from build123d import *

# Parameters (mm, degrees)
BOSS_EXTRUDE1_DEPTH            = 3.175
SKETCH2_W                      = 31.75
SKETCH2_H                      = 82.55
CUT_EXTRUDE1_DEPTH             = 4.175
FILLET1_R                      = 3.175
F_1_4_0_25_DIAMETER_HOLE1_D    = 6.35
F_1_4_CLEARANCE_HOLE1_D        = 6.7564
F_5_16_0_3125_DIAMETER_HOLE1_D = 7.9375
CUT_EXTRUDE2_DEPTH             = 4.175
FILLET2_R                      = 6.35
SKETCH12_W                     = 31.75
SKETCH12_H                     = 50.8
CUT_EXTRUDE3_DEPTH             = 4.175
FILLET3_R                      = 3.175


with BuildPart() as part:
    # Sketch1 → Boss-Extrude1 (new body)
    with BuildSketch(Plane(origin=(0, 0, 0), x_dir=(1, 0, 0), z_dir=(0, 1, 0))):
        with BuildLine():
            Line((-260.839523021, 465.231358695), (-482.578348021, 61.34030281))
            Line((-482.578348021, 61.34030281), (-458.5319125, 48.13865281))
            ThreePointArc((-458.5319125, 48.13865281), (-449.57100781, 39.462418136), (-446.278, 27.432))
            Line((-446.278, 27.432), (-446.278, 0))
            Line((-446.278, 0), (446.278, 0))
            Line((446.278, 0), (446.278, 27.432))
            ThreePointArc((446.278, 27.432), (449.57100781, 39.462418136), (458.5319125, 48.13865281))
            Line((458.5319125, 48.13865281), (482.578348021, 61.34030281))
            Line((482.578348021, 61.34030281), (260.839523021, 465.231358695))
            Line((260.839523021, 465.231358695), (236.7930875, 452.029708695))
            ThreePointArc((236.7930875, 452.029708695), (213.394581864, 452.407369315), (201.803, 472.736361505))
            Line((201.803, 472.736361505), (201.803, 500.168361505))
            Line((201.803, 500.168361505), (-201.803, 500.168361505))
            Line((-201.803, 500.168361505), (-201.803, 472.736361505))
            ThreePointArc((-201.803, 472.736361505), (-213.394581864, 452.407369315), (-236.7930875, 452.029708695))
            Line((-236.7930875, 452.029708695), (-260.839523021, 465.231358695))
        make_face()
    extrude(amount=BOSS_EXTRUDE1_DEPTH)

    # Sketch2 → Cut-Extrude1 (cut, through all)
    with BuildSketch(Plane(origin=(0, 3.175, 0), x_dir=(1, 0, 0), z_dir=(0, 1, 0))):
        with Locations((-304.8, 41.275)):
            Rectangle(SKETCH2_W, SKETCH2_H)
        with Locations((304.8, 41.275)):
            Rectangle(SKETCH2_W, SKETCH2_H)
    extrude(amount=-CUT_EXTRUDE1_DEPTH, mode=Mode.SUBTRACT)

    # Fillet1
    fillet1_edges = [part.edges().sort_by_distance(p)[0] for p in [
        (-288.925, 1.5875, -82.55),
        (-288.925, 1.5875, 0),
        (-320.675, 1.5875, 0),
        (-320.675, 1.5875, -82.55),
        (288.925, 1.5875, 0),
        (288.925, 1.5875, -82.55),
        (320.675, 1.5875, -82.55),
        (320.675, 1.5875, 0),
    ]]
    fillet(fillet1_edges, radius=FILLET1_R)

    # 1/4 (0.25) Diameter Hole1 (through all)
    with Locations(Plane(origin=(0, 3.175, 0), x_dir=(1, 0, 0), z_dir=(0, 1, 0))):
        with Locations((-465.394777961, 66.250083744), (-272.870715461, 416.927268429), (-177.8, 487.468361505), (465.394777961, 66.250083744), (272.870715461, 416.927268429), (177.8, 487.468361505)):
            Hole(F_1_4_0_25_DIAMETER_HOLE1_D / 2)

    # 1/4 Clearance Hole1 (through all)
    with Locations(Plane(origin=(0, 3.175, 0), x_dir=(1, 0, 0), z_dir=(0, 1, 0))):
        with Locations((0, 224.282), (-376.682, 50.8), (-185.674, 398.526), (376.682, 50.8), (185.674, 398.526)):
            Hole(F_1_4_CLEARANCE_HOLE1_D / 2)

    # 5/16 (0.3125) Diameter Hole1 (through all)
    with Locations(Plane(origin=(0, 3.175, 0), x_dir=(1, 0, 0), z_dir=(0, 1, 0))):
        with Locations((-254, 50.8), (-114.3, 449.368361505), (254, 50.8), (114.3, 449.368361505)):
            Hole(F_5_16_0_3125_DIAMETER_HOLE1_D / 2)

    # Sketch11 → Cut-Extrude2 (cut, through all)
    with BuildSketch(Plane(origin=(0, 3.175, 0), x_dir=(1, 0, 0), z_dir=(0, 1, 0))):
        Polygon((0, 256.032), (159.899523893, 417.618361505), (-159.899523893, 417.618361505), align=None)
    extrude(amount=-CUT_EXTRUDE2_DEPTH, mode=Mode.SUBTRACT)

    # Fillet2
    fillet2_edges = [part.edges().sort_by_distance(p)[0] for p in [
        (0, 1.5875, -256.032),
        (-159.899523893, 1.5875, -417.618361505),
        (159.899523893, 1.5875, -417.618361505),
    ]]
    fillet(fillet2_edges, radius=FILLET2_R)

    # Sketch12 → Cut-Extrude3 (cut, through all)
    with BuildSketch(Plane(origin=(0, 3.175, 0), x_dir=(1, 0, 0), z_dir=(0, 1, 0))):
        with Locations((0, 474.768361505)):
            Rectangle(SKETCH12_W, SKETCH12_H)
    extrude(amount=-CUT_EXTRUDE3_DEPTH, mode=Mode.SUBTRACT)

    # Fillet3
    fillet3_edges = [part.edges().sort_by_distance(p)[0] for p in [
        (-15.875, 1.5875, -449.368361505),
        (-15.875, 1.5875, -500.168361505),
        (15.875, 1.5875, -500.168361505),
        (15.875, 1.5875, -449.368361505),
    ]]
    fillet(fillet3_edges, radius=FILLET3_R)


solid = part.part
CAD build for the part. Positions are in the model's coordinates, mm. A direction names the side the tool comes from. Give positions to 0.01 mm unless a question says otherwise; leave off trailing zeros. Loops run counter-clockwise (first coordinate to the right, second up) from the corner with the lowest first, then second, coordinate; pieces in that order, holes last. Notation, with made-up numbers: M 18,-11 L 33,-11 A31 cw 33,18 Z; hole C 69.5,-28 d4. An arc over 180 degrees is marked long. Answer in a Markdown table with one row per item. Add a question column.
Item 1: Band-saw the part on C-C on y = 0.6. Give the number of separate pieces and of enclosed holes in the cut face, then the cut area to 3 significant figures.
Item 2: Mould opens along X. For faces 1 (the face through (213.691, 1.565, -452.235)), 2 (the face through (-7, 3.175, -198)), 3 (the face through (-213.101, 1.565, -452.584)), 4 (the face through (373.26, 1.57, -260.46)) say: +X half, -X half, draft (parallel to the pull), parting line (faces both ways), or undercut.
Item 3: Tool access for faces 5 (the face through (-7, 0, -198)), 6 (the face through (-77.868, 1.61, -334.721)): list every direction of +Z, -Z, +X, -X, +Y, -Y with a clear straight run to the whole face (end or side of a thin tool).
Item 4: Drop flat-ended pins along their axis: P1, Ø1.6, axis at x = -298.5, y = 2, coming from the +Z side; P2, Ø1.6, axis at y = 1.5, z = -484, coming from the +X side. Give the stop position or say it passes through.
Item 5: Band-saw the part on B-B on x = -34. Give the cut face in (y, z) (3 decimals), then the cut area to 3 significant figures.
Item 6: Band-saw the part on A-A on z = -279. Give the cut face in (x, y) (3 decimals).
Item 7: Probe probe 1 along Z at (x, y) = (45, 2.75); probe 2 along Z at (x, y) = (114.3, 2.3); probe 3 along X at (y, z) = (1.35, -390.5). List the from-to ranges inside material, lowest first.
Item 8: Band-saw the part on D-D on z = -433.5. Give the cut face in (x, y) (3 decimals), then the cut area to 3 significant figures.
Reply:
| question | item | result |
|---|---|---|
| 1 | separate pieces | 1 |
| 1 | enclosed holes | 16 |
| 1 | area | 336,000 mm^2 |
| 2 | face 1 | undercut |
| 2 | face 2 | draft |
| 2 | face 3 | undercut |
| 2 | face 4 | +X half |
| 3 | face 5 | +Z, -Z, +X, -X, -Y |
| 3 | face 6 | +Y, -Y |
| 4 | P1 | stops at z = -82.55 |
| 4 | P2 | stops at x = 201.8 |
| 5 | outline | M 0,-500.168 L 3.175,-500.168 L 3.175,-417.618 L 0,-417.618 Z; M 0,-290.391 L 3.175,-290.391 L 3.175,0 L 0,0 Z |
| 5 | area | 1,180 mm^2 |
| 6 | outline | M -363.082,0 L -22.728,0 L -22.728,3.175 L -363.082,3.175 Z; M 22.728,0 L 363.082,0 L 363.082,3.175 L 22.728,3.175 Z |
| 7 | probe 1 | z = -500.17 to -417.62, -301.51 to 0 |
| 7 | probe 2 | z = -500.17 to -453.34, -445.4 to -417.62, -371.54 to 0 |
| 7 | probe 3 | x = -301.87 to -133.06, 133.06 to 301.87 |
| 8 | outline | M -278.26,0 L 278.26,0 L 278.26,3.175 L -278.26,3.175 Z |
| 8 | area | 1,770 mm^2 |
